```python
from build123d import *

# Parameters (mm, degrees)
F1_DEPTH = 10.16
F3_D     = 6.35


with BuildPart() as f1:
    # F0 (on Right) → F1 (new body)
    with BuildSketch(Plane.YZ):
        Polygon((-77.474721, 10.765259), (-103.973828, 0), (-112.688757, -4.140489), (-156.410038, -25.118949), (-138.453096, -24.566885), (-100.977682, -17.942108), (-69.748186, -11.869396), (-39.299428, -5.244619), (-22.903949, -6.900813), (1.298919, -5.244619), (9.106293, -6.348748), (16.913667, -22.358626), (5.202606, -39.472636), (-6.508455, -59.346966), (2.860397, -75.908907), (41.89726, -75.356841), (30.186206, -72.59652), (37.212841, -71.492389), (48.923902, -60.451094), (48.923902, -57.690769), (35.651371, -59.346966), (24.721041, -66.523813), (17.694414, -60.451094), (17.694414, -53.826321), (24.721041, -40.576763), (37.212841, -30.639596), (54.389074, -12.973526), (52.046858, -1.93223), (63.757919, -0.828101), (91.864459, -11.317331), (98.891109, -13.52559), (98.891109, -22.358626), (91.864459, -30.639596), (90.302989, -26.22308), (83.276354, -32.847855), (90.302989, -35.056114), (98.891109, -33.399921), (104.356274, -30.639596), (113.725118, -14.077655), (104.356274, -6.348748), (82.495622, 2.484288), (79.372667, 8.557), (98.110363, 19.598294), (105.917737, 30.639591), (107.47923, 41.680887), (116.848074, 47.753599), (130.901337, 51.065989), (142.612413, 53.274248), (145.735353, 59.346959), (144.954622, 63.763477), (134.024292, 68.73206), (85.936449, 68.73206), (79.311676, 65.971732), (74.343085, 57.1387), (68.270378, 26.775137), (56.124948, 32.295786), (39.010942, 32.295786), (27.417587, 32.295786), (13.063898, 26.775137), (0, 21.254489), (-22.820309, 21.254489), (-53.735938, 17.942103), align=None)
    extrude(amount=F1_DEPTH)

    # F3 (through all)
    with Locations(Plane.YZ.offset(10.16)):
        with Locations((105.92816, 61.003152)):
            Hole(F3_D / 2)


solid = f1.part
```
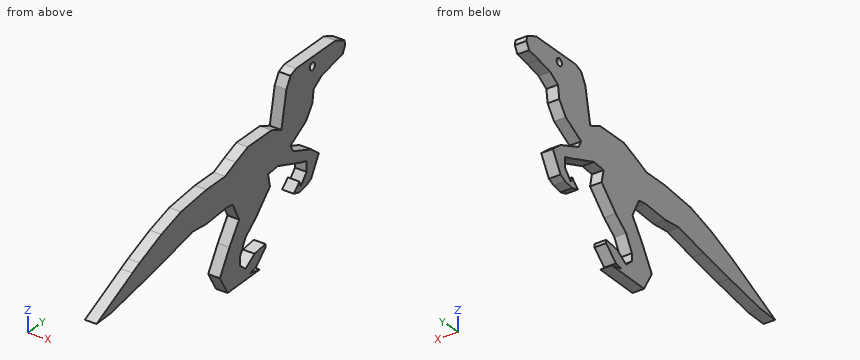
Check sheet for the modelled part. Datum: model origin and axes. Units: mm. Give positions to 0.01 mm unless a question says otherwise; leave off trailing zeros. Order: outer loops, then holes, each group sorted by start corner. A loop starts at its lowest first (then second) coordinate and runs counter-clockwise, first axis right, second up. Notation, with made-up numbers: (-9, 75.5) -> (-2, 75.5) arc R13 cw to (-2, 86.5) -> close; hole circle Ø8 at (28.25, 64.5). An arc over 180 degrees is marked (long way). Use CSV: the item, a comma, the result in double quotes. Start each with the question number.
1) Sectioned sample at B-B, the plane y = -18.5. Record the boundary of the cut face in (x, z), plus the area to 3 significant figures.
2) Go/stop test with flat-tipped pins: P1, Ø10, axis at y = 105.93, z = 61, coming from the -X side; P2, Ø1.4, axis at x = 5, z = -59.5, coming from the +Y side; P3, Ø1, axis at x = 3.5, z = 42, coming from the +Y side; P4, Ø4.5, axis at x = 5.5, z = -19.5, coming from the -Y side. Record where each tip stops, or that it passes through.
3) Sectioned sample at A-A, the plane y = -50. Record the boundary of the cut face in (x, z), plus the area to 3 significant figures.
4) Material ranges on line 1 (Z direction, x = 2, y = 84.5); line 2 (Z direction, x = 0.5, y = 94); line 3 (Z direction, x = 1, y = 80), recorded low to high. Write a range as from..to.
Recorded:
1,outline,"(0, -6.6) -> (10.16, -6.6) -> (10.16, 21.25) -> (0, 21.25) -> close"
1,area,"283 mm2"
2,P1,"x = 0"
2,P2,"y = 48.92"
2,P3,"y = 108.74"
2,P4,"y = -149.39"
3,outline,"(0, -7.57) -> (10.16, -7.57) -> (10.16, 18.34) -> (0, 18.34) -> close"
3,area,"263 mm2"
4,line 1,"-33.23..-31.69, -8.57..1.67, 11.58..68.13"
4,line 2,"-34.34..-28.12, -11.99..-2.16, 17.18..68.73"
4,line 3,"-6.89..7.34, 8.93..66.26"
